Can you work these out from the model? Positions are in its coordinate system, mm. A direction names the side the tool comes from. Give positions to 0.01 mm unless a question says otherwise; leave off trailing zeros. Order: outer loops, then holes, each group sorted by start corner. A loop starts at its lowest first (then second) coordinate and runs counter-clockwise, first axis right, second up. Notation, with made-up numbers: (59, 59) - (97, 59) arc R34 cw to (97, 98) - close; hole circle Ø8 at (20.5, 42). An arc over 180 degrees is marked (long way). One line per question, with ' | ' between items.
```python
from build123d import *

# Parameters (mm, degrees)
BOSS_EXTRUDE1_DEPTH = 7
BOSS_EXTRUDE2_DEPTH = 13
SKETCH3_R           = 2.5
BOSS_EXTRUDE3_DEPTH = 10


with BuildPart() as part:
    # Sketch1 → Boss-Extrude1 (new body)
    with BuildSketch(Plane.XY):
        with BuildLine():
            Line((-2.875, 1.25), (2.875, 1.25))
            ThreePointArc((2.875, 1.25), (4.125, 0), (2.875, -1.25))
            Line((2.875, -1.25), (-2.875, -1.25))
            ThreePointArc((-2.875, -1.25), (-4.125, 0), (-2.875, 1.25))
        make_face()
    extrude(amount=BOSS_EXTRUDE1_DEPTH)

    # Sketch2 → Boss-Extrude2 (add)
    with BuildSketch(Plane.XY.offset(7)):
        with BuildLine():
            Line((-3.5, 3), (3.5, 3))
            ThreePointArc((3.5, 3), (6.5, 0), (3.5, -3))
            Line((3.5, -3), (-3.5, -3))
            ThreePointArc((-3.5, -3), (-6.5, 0), (-3.5, 3))
        make_face()
    extrude(amount=BOSS_EXTRUDE2_DEPTH)

    # Sketch3 → Boss-Extrude3 (add)
    with BuildSketch(Plane.XY.offset(20)):
        Circle(SKETCH3_R)
    extrude(amount=BOSS_EXTRUDE3_DEPTH)


solid = part.part
```
(1) Imagine slicing it at B-B (y = 0). List the corners of the cut face in (x, z) for me (3 decimals).
Answer below:
outline: (-6.5, 7) - (-4.125, 7) - (-4.125, 0) - (4.125, 0) - (4.125, 7) - (6.5, 7) - (6.5, 20) - (2.5, 20) - (2.5, 30) - (-2.5, 30) - (-2.5, 20) - (-6.5, 20) - close
(2) Imagine slicing it at D-D (z = 14.5). List the corners of the cut face in (x, y) for me, and give its area (3 significant figures).
Answer below:
outline: (-3.5, -3) - (3.5, -3) arc R3 ccw to (3.5, 3) - (-3.5, 3) arc R3 ccw to start | area: 70.3 mm^2
(3) If I drill on line 1 (Z direction, x = 3.75, y = -0.35); line 2 (Y direction, x = -1.5, z = 5.25); line 3 (Z direction, x = -3, y = -2.15), over which ranges is the centre line in solid material (lowest first)?
Answer below:
line 1: 0 to 20 | line 2: -1.25 to 1.25 | line 3: 7 to 20
(4) Will these pins go through, and if not, where does the flat tip stop? pin 1 (1 mm diameter, centred on x = 3.5, y = -2, fed in from -Z); pin 2 (1.7 mm diameter, centred on x = -1, z = 2, fed in from -Y); pin 3 (5 mm diameter, centred on x = 1.5, z = 23, fed in from -Y).
Answer below:
pin 1: z = 7 | pin 2: y = -1.25 | pin 3: y = -2.5
(5) Imagine slicing it at C-C (z = 21.25). List the corners of the cut face in (x, y) for me.
Answer below:
outline: circle Ø5 at (0, 0)
(6) Imagine slicing it at A-A (x = 0). List the corners of the cut face in (y, z) for me.
Answer below:
outline: (-3, 7) - (-1.25, 7) - (-1.25, 0) - (1.25, 0) - (1.25, 7) - (3, 7) - (3, 20) - (2.5, 20) - (2.5, 30) - (-2.5, 30) - (-2.5, 20) - (-3, 20) - close
(7) On a 3-axis mill with a long thin cutter (end or side, diameter ignored), from which of +Z, -Z, +X, -X, +Y, -Y can I reach the whole of each face in a straight line? I mean faces 1 (the face through (-4.125, -0.027, 3.451)), 2 (the face through (-0.54, -2.44, 24.93)), 3 (the face through (4.125, 0.027, 3.451)), 4 (the face through (0, -1.25, 3)), 5 (the face through (0, 1.25, 3)). Say none if no direction works.
Answer below:
face 1: -Z, -X | face 2: +Z | face 3: -Z, +X | face 4: -Z, +X, -X, -Y | face 5: -Z, +X, -X, +Y
